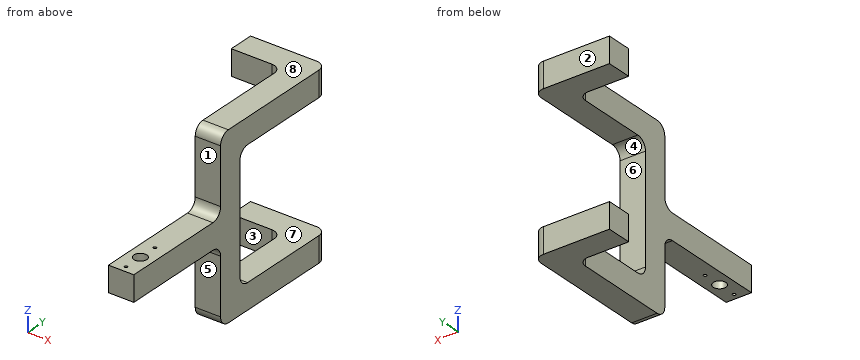
```python
from build123d import *

# Parameters (mm, degrees)
ESQUISSE1_W        = 10
ESQUISSE1_H        = 55
ESQUISSE1_R        = 2.5
ESQUISSE1_R_2      = 0.5
BOSS_EXTRU_1_DEPTH = 10
BOSS_EXTRU_2_DEPTH = 10
ESQUISSE5_W        = 10
ESQUISSE5_H        = 10
BOSS_EXTRU_3_DEPTH = 20
CONG_1_R           = 4
D_GAGEMENT_M11_D   = 1.2


with BuildPart() as part:
    # Esquisse1 → Boss.-Extru.1 (new body)
    with BuildSketch(Plane.XY):
        with Locations((9, 27.5)):
            Rectangle(ESQUISSE1_W, ESQUISSE1_H)
        with Locations((9, 10)):
            Circle(ESQUISSE1_R, mode=Mode.SUBTRACT)
        with Locations((9, 17.5)):
            Circle(ESQUISSE1_R_2, mode=Mode.SUBTRACT)
        with Locations((9, 2.5)):
            Circle(ESQUISSE1_R_2, mode=Mode.SUBTRACT)
    extrude(amount=BOSS_EXTRU_1_DEPTH)

    # Esquisse4 → Boss.-Extru.2 (add)
    with BuildSketch(Plane(origin=(14, 0, 0), x_dir=(0, 0, -1), z_dir=(1, 0, 0))):
        Polygon((-30, 55), (20, 55), (20, 100), (30, 100), (30, 45), (-40, 45), (-40, 100), (-30, 100), align=None)
    extrude(amount=-BOSS_EXTRU_2_DEPTH)

    # Esquisse5 → Boss.-Extru.3 (add)
    with BuildSketch(Plane.ZY.offset(-4)):
        with Locations((-25, 95)):
            Rectangle(ESQUISSE5_W, ESQUISSE5_H)
        with Locations((35, 95)):
            Rectangle(ESQUISSE5_W, ESQUISSE5_H)
    extrude(amount=BOSS_EXTRU_3_DEPTH)

    # Congé1
    cong_1_edges = [part.edges().sort_by_distance(p)[0] for p in [
        (9, 45, 0),
        (9, 45, -30),
        (14, 100, -25),
        (9, 55, -20),
        (9, 45, 10),
        (9, 45, 40),
        (9, 55, 30),
        (14, 100, 35),
        (4, 90, -25),
        (4, 90, 35),
    ]]
    fillet(cong_1_edges, radius=CONG_1_R)

    # Dégagement M11 (through all)
    with Locations(Plane.XY.offset(10)):
        with Locations((9, 17.5), (9, 2.5)):
            Hole(D_GAGEMENT_M11_D / 2)


solid = part.part
```
Input: part model. Units: mm. Frame: model coordinates. Face numbers are marked on the shaded views. A direction names the side the tool comes from. Give positions to 0.01 mm unless a question says otherwise; leave off trailing zeros. Order: outer loops, then holes, each group sorted by start corner. A loop starts at its lowest first (then second) coordinate and runs counter-clockwise, first axis right, second up. Notation, with made-up numbers: M 64.25,3.5 L 110.25,3.5 A11 ccw 110.25,24.5 Z; hole C 70.5,72.5 d2. An arc over 180 degrees is marked long. Return JSON: item names as keys, results as strings.
1) Section query A-A on y = 10. Output: boundary loops of the cut face in (x, z), and give its area (3 significant figures).
Taken from the geometry:
{"outline": "M 4,0 L 6.5,0 L 6.5,10 L 4,10 Z; M 11.5,0 L 14,0 L 14,10 L 11.5,10 Z", "area": "50.0 mm2"}
2) Section query D-D on z = -24.5. Output: boundary loops of the cut face in (x, y), and give its area (3 significant figures).
Taken from the geometry:
{"outline": "M -16,90 L 0,90 A4 cw 4,86 L 4,45 L 14,45 L 14,96 A4 ccw 10,100 L -16,100 Z", "area": "750 mm2"}
3) Section query B-B on x = -6.25. Output: boundary loops of the cut face in (y, z), and give its area (3 significant figures).
Taken from the geometry:
{"outline": "M 90,-30 L 100,-30 L 100,-20 L 90,-20 Z; M 90,30 L 100,30 L 100,40 L 90,40 Z", "area": "200 mm2"}
4) Section query C-C on z = 7.5. Output: boundary loops of the cut face in (x, y).
Taken from the geometry:
{"outline": "M 4,0 L 14,0 L 14,55 L 4,55 Z; hole C 9,10 d5; hole C 9,2.5 d1.2; hole C 9,17.5 d1.2"}
5) Mould query, pull axis Z, two halves, no side actions, for the marked faces 5, 6, 7 and 8. Classes: released by +Z, released by -Z, zero draft, split by the parting line, or undercut.
Taken from the geometry:
{"face 5": "zero draft", "face 6": "undercut", "face 7": "undercut", "face 8": "released by +Z"}
6) Contact query for flat-ended pins moving along their axis: pin 1 (1.6 mm diameter, centred on x = 9, y = 17.5, fed in from +Z); pin 2 (1.5 mm diameter, centred on x = 8, z = -13, fed in from -Y); pin 3 (8 mm diameter, centred on x = 10, z = 3.5, fed in from +Y). Output: stop coordinate, or through.
Taken from the geometry:
{"pin 1": "stops at z = 10", "pin 2": "stops at y = 45", "pin 3": "stops at y = 55"}
7) Line query: L1, parallel to Y at x = 9, z = 7.25; L2, parallel to Z at x = -1.25, y = 94.5; L3, parallel to Z at x = 7.75, y = 7. Output: solid intervals per line, ascending. Write a range as [from, to].
Taken from the geometry:
{"L1": "y = [0, 1.9], [3.1, 7.5], [12.5, 16.9], [18.1, 55]", "L2": "z = [-30, -20], [30, 40]", "L3": "z = [0, 10]"}
8) Access query for the marked faces 1, 2, 3 and 4. Directions: +Z, -Z, +X, -X, +Y, -Y. A direction counts if a zero-diameter tool reaches every point of the face in a straight line with its end or side. Return the directions, or none.
Taken from the geometry:
{"face 1": "+Z, +X, -X, -Y", "face 2": "+Z, -Z, +X, -X, +Y", "face 3": "+Z, -Z, -X, -Y", "face 4": "+X, -X, +Y"}
